Autodesk Inventor part; units mm, degrees
ref_plane "YZ Plane" through (0, 0, 0) normal (1, 0, 0) x (0, 1, 0)
ref_plane "XZ Plane" through (0, 0, 0) normal (0, 1, 0) x (-1, 0, 0)
ref_plane "XY Plane" through (0, 0, 0) normal (0, 0, 1) x (1, 0, 0)
sketch "Sketch1" plane through (0, 0, 0) normal (0, 1, 0) x (-1, 0, 0)
  line L0 (26.5, 16.5) -> (-26.5, 16.5) construction
  line L1 (-26.5, 16.5) -> (-26.5, -16.5) construction
  line L2 (-26.5, -16.5) -> (26.5, -16.5) construction
  line L3 (26.5, -16.5) -> (26.5, 16.5) construction
  line L4 (26.5, -16.5) -> (-26.5, 16.5) construction
  circle A0 centre (26.5, 16.5) radius 1
  circle A1 centre (26.5, -16.5) radius 1
  circle A2 centre (-26.5, 16.5) radius 1
  circle A3 centre (-26.5, -16.5) radius 1
  circle A4 centre (26.5, 16.5) radius 3.75
  circle A5 centre (26.5, -16.5) radius 3.75
  circle A6 centre (-26.5, -16.5) radius 3.75
  circle A7 centre (-26.5, 16.5) radius 3.75
  point P0 (0, 0)
  point P1 (0, 0)
  dimension "d0" = 33
  dimension "d1" = 53
  dimension "d2" = 2
  dimension "d3" = 7.5
extrude "Extrusion1" add sketch "Sketch1" along normal blind 7.5
sketch "Sketch2" plane through (0, 0, 0) normal (0, 1, 0) x (-1, 0, 0)
  line L0 (37.5, -25) -> (-37.5, -25)
  line L1 (-37.5, -25) -> (-37.5, 25)
  line L2 (-37.5, 25) -> (37.5, 25)
  line L3 (37.5, 25) -> (37.5, -25)
  line L4 (37.5, 25) -> (-37.5, -25) construction
  line L5 (35.5, -19) -> (35.5, 19)
  line L6 (-35.5, 19) -> (-35.5, -19)
  circle A0 centre (-26.5, -16.5) radius 1
  circle A1 centre (26.5, -16.5) radius 3.75
  circle A2 centre (26.5, 16.5) radius 3.75
  circle A3 centre (-26.5, 16.5) radius 3.75
  arc A4 (35.5, -19) -> (31.5, -23) centre (35.5, -23) ccw
  arc A5 (31.5, 23) -> (35.5, 19) centre (35.5, 23) ccw
  arc A6 (-35.5, 19) -> (-31.5, 23) centre (-35.5, 23) ccw
  arc A7 (-31.5, -23) -> (-35.5, -19) centre (-35.5, -23) ccw
  line L7 (-31.5, -23) -> (31.5, -23)
  line L8 (31.5, 23) -> (-31.5, 23)
  point P0 (0, 0)
  point P1 (0, 0)
  dimension "d6" = 75
  dimension "d10" = 50
  dimension "d11" = 2
  dimension "d129" = 4
  dimension "d132" = 2
  dimension "d133" = 2
  dimension "d134" = 2
extrude "Extrusion7" add sketch "Sketch2" against normal blind 2 contours L0 L1 L2 L3 | A4 L7 A7 L6 A6 L8 A5 L5 | A0 | A1 | A2 | A3
extrude "Extrusion8" add sketch "Sketch2" along normal blind 30 contours L0 L1 L2 L3
sketch "Sketch6" plane through (0, 30, 0) normal (0, 1, 0) x (1, 0, 0)
  circle A0 centre (-35.5, 23) radius 1
  line L0 (-32.6716, 23) -> (32.6716, 23)
  line L1 (-35.5, -20.1716) -> (-35.5, 20.1716)
  circle A1 centre (35.5, 23) radius 1
  circle A2 centre (35.5, -23) radius 1
  circle A3 centre (-35.5, -23) radius 1
  line L2 (35.5, 20.1716) -> (35.5, -20.1716)
  line L3 (32.6716, -23) -> (-32.6716, -23)
  point P0 (0, 0)
  dimension "d24" = 2
extrude "Extrusion9" cut sketch "Sketch6" against normal blind 10
fillet "Fillet2" radius 2 4 edges at (-37.5, 14, -25) (-37.5, 14, 25) (37.5, 14, 25) (37.5, 14, -25)
fillet "Fillet3" radius 2 8 edges at (32.6716, 0, 20.1716) (35.5, 0, 0) (32.6716, 0, -20.1716) (0, 0, -23) (-32.6716, 0, -20.1716) (-35.5, 0, 0) (-32.6716, 0, 20.1716) (0, 0, 23)
properties part number "Enclosure"
Geometry: final body of the model. Coordinates: model frame, mm. A direction names the side the tool comes from. Round coordinates to 2 decimals unless told otherwise and drop trailing zeros. Loops run counter-clockwise (first coordinate to the right, second up) from the corner with the lowest first, then second, coordinate; pieces in that order, holes last. Notation, with made-up numbers: (7.25, 71.5) -> (57.25, 71.5) arc R13 ccw to (57.25, 77.5) -> close; hole circle Ø7 at (87.25, 33.5). An arc over 180 degrees is marked (long way). Write each question's results on one line, items separated by ' | '.
Item 1: Cut plane B-B on z = 16.5. Return the cut outline in (x, y), and give its area (3 significant figures).
Answers below:
outline: (-37.5, -2) -> (37.5, -2) -> (37.5, 30) -> (35.5, 30) -> (35.5, 2) arc R2 cw to (33.5, 0) -> (30.25, 0) -> (30.25, 7.5) -> (27.5, 7.5) -> (27.5, 0) -> (25.5, 0) -> (25.5, 7.5) -> (22.75, 7.5) -> (22.75, 0) -> (-22.75, 0) -> (-22.75, 7.5) -> (-25.5, 7.5) -> (-25.5, 0) -> (-27.5, 0) -> (-27.5, 7.5) -> (-30.25, 7.5) -> (-30.25, 0) -> (-33.5, 0) arc R2 cw to (-35.5, 2) -> (-35.5, 30) -> (-37.5, 30) -> close | area: 354 mm²
Item 2: Line query: probe 1 along Z at (x, y) = (-26.5, 4); probe 2 along X at (y, z) = (2.5, 6); probe 3 along Z at (x, y) = (9, 9.5). Output: solid intervals per line, ascending. Write a range as [from, to].
Answers below:
probe 1: z = [-25, -23], [-20.25, -17.5], [-15.5, -12.75], [12.75, 15.5], [17.5, 20.25], [23, 25] | probe 2: x = [-37.5, -35.5], [35.5, 37.5] | probe 3: z = [-25, -23], [23, 25]
Item 3: Cut plane D-D on x = 26.5. Return the cut outline in (y, z).
Answers below:
outline: (-2, -25) -> (30, -25) -> (30, -23) -> (2, -23) arc R2 cw to (0, -21) -> (0, -20.25) -> (7.5, -20.25) -> (7.5, -17.5) -> (0, -17.5) -> (0, -15.5) -> (7.5, -15.5) -> (7.5, -12.75) -> (0, -12.75) -> (0, 12.75) -> (7.5, 12.75) -> (7.5, 15.5) -> (0, 15.5) -> (0, 17.5) -> (7.5, 17.5) -> (7.5, 20.25) -> (0, 20.25) -> (0, 21) arc R2 cw to (2, 23) -> (30, 23) -> (30, 25) -> (-2, 25) -> close
Item 4: Set-up query: faces 1 (the face through (0.44, 0.6, 22.43)), 2 (the face through (37.5, 14, 0)). Return all of +Z, -Z, +X, -X, +Y, -Y with unobstructed straight access to the full face (end or side cutting, diameter ignored); none if empty.
Answers below:
face 1: +Y | face 2: +Z, -Z, +X, +Y, -Y
Item 5: Pin query (flat end, axial travel): pin 1 Ø4 at (x, z) = (26, -16) entering from +Y; pin 2 Ø4 at (x, z) = (23.5, 10) entering from +Y; pin 3 Ø0.6 at (x, z) = (-35, -23) entering from +Y; pin 4 Ø3 at (x, z) = (35.5, -23) entering from +Y. Return the tip coordinate at first contact, or that it passes through.
Answers below:
pin 1: stops at y = 7.5 | pin 2: stops at y = 0 | pin 3: stops at y = 20 | pin 4: stops at y = 30
Item 6: Cut plane A-A on y = 21. Return the cut outline in (x, z).
Answers below:
outline: (-37.5, -23) arc R2 ccw to (-35.5, -25) -> (35.5, -25) arc R2 ccw to (37.5, -23) -> (37.5, 23) arc R2 ccw to (35.5, 25) -> (-35.5, 25) arc R2 ccw to (-37.5, 23) -> close; hole circle Ø2 at (-35.5, -23); hole circle Ø2 at (-35.5, 23); hole (-35.5, -19) arc R4 cw to (-31.5, -23) -> (31.5, -23) arc R4 cw to (35.5, -19) -> (35.5, 19) arc R4 cw to (31.5, 23) -> (-31.5, 23) arc R4 cw to (-35.5, 19) -> close; hole circle Ø2 at (35.5, -23); hole circle Ø2 at (35.5, 23)
Item 7: Pull-direction query (Z, two-part tool) for faces 3 (the face through (34.93, 0.6, -0.27)), 4 (the face through (-36.93, 14.22, 24.4)), 5 (the face through (1, -2, 0)); classes: pulls with the +Z half, pulls with the -Z half, needs draft (parallel to the pull), parting line crosses it, or undercut.
Answers below:
face 3: undercut | face 4: pulls with the +Z half | face 5: needs draft
Item 8: Cut plane C-C on y = 11.5. Return the cut outline in (x, z), and give its area (3 significant figures).
Answers below:
outline: (-37.5, -23) arc R2 ccw to (-35.5, -25) -> (35.5, -25) arc R2 ccw to (37.5, -23) -> (37.5, 23) arc R2 ccw to (35.5, 25) -> (-35.5, 25) arc R2 ccw to (-37.5, 23) -> close; hole (-35.5, -19) arc R4 cw to (-31.5, -23) -> (31.5, -23) arc R4 cw to (35.5, -19) -> (35.5, 19) arc R4 cw to (31.5, 23) -> (-31.5, 23) arc R4 cw to (-35.5, 19) -> close | area: 531 mm²
